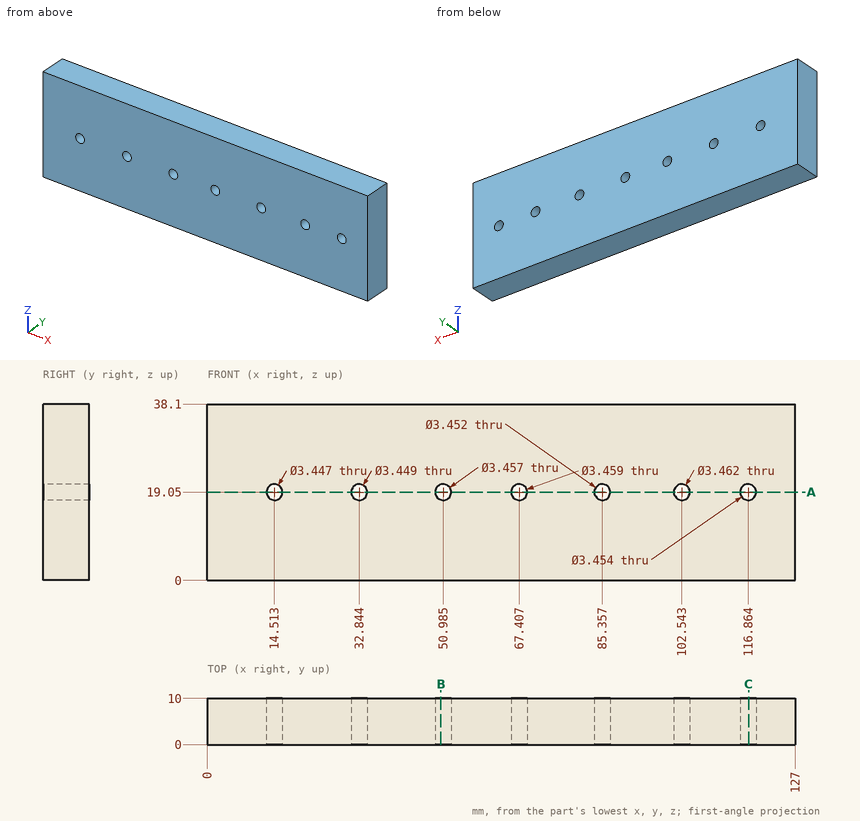
Here's the drawing with two shaded views (mm, measured from the low corner). I have some questions. Round coordinates to 2 decimals unless told otherwise and drop trailing zeros. Write each loop counter-clockwise with the first axis right and the second up, starting at its lowest first coordinate (ties: lowest second). Pieces come first, ordered by that corner, then holes.
(1) Suppose I cut it at C-C on x = 117. Write out the boundary of the cut face in (y, z).
Findings below:
outline: (0, 0) - (10, 0) - (10, 17.33) - (0, 17.33) - close; (0, 20.77) - (10, 20.77) - (10, 38.1) - (0, 38.1) - close
(2) Suppose I cut it at B-B on x = 50.5. Write out the boundary of the cut face in (y, z), and give its area (3 significant figures).
Findings below:
outline: (0, 0) - (10, 0) - (10, 17.39) - (0, 17.39) - close; (0, 20.71) - (10, 20.71) - (10, 38.1) - (0, 38.1) - close
area: 348 mm2
(3) Suppose I cut it at A-A on z = 19.05. State how many separate pieces and enclosed holes the cut face has, and give its area (3 significant figures).
Findings below:
separate pieces: 8
enclosed holes: 0
area: 1,030 mm2
(4) If I drill on probe 1 along Z at (x, y) = (14.5, 6.5); probe 2 along Z at (x, y) = (51.5, 9), over which ranges is the centre line in solid material (lowest first)?
Findings below:
probe 1: z = 0 to 17.33, 20.77 to 38.1
probe 2: z = 0 to 17.4, 20.7 to 38.1
